```python
from build123d import *

# Parameters (mm, degrees)
SKETCH1_R           = 3.5
BOSS_EXTRUDE6_DEPTH = 5
CUT_EXTRUDE5_DEPTH  = 14.035691085
FILLET3_R           = 2
SKETCH3_R           = 3.5
BOSS_EXTRUDE9_DEPTH = 3


with BuildPart() as part:
    # Sketch1 → Boss-Extrude6 (new body)
    with BuildSketch(Plane.XY):
        with BuildLine():
            Line((1.138484568, -6.230529798), (82.159951164, -6.236480839))
            ThreePointArc((82.159951164, -6.236480839), (86.188937946, -4.567966564), (87.858044062, -0.539224931))
            Line((87.858044062, -0.539224931), (87.858163632, 1.088682041))
            ThreePointArc((87.858163632, 1.088682041), (86.189649357, 5.117668823), (82.160907724, 6.786774939))
            Line((82.160907724, 6.786774939), (8.344270935, 6.792196785))
            Line((8.344270935, 6.792196785), (-81.443742997, 6.79879173))
            ThreePointArc((-81.443742997, 6.79879173), (-85.472729779, 5.130277455), (-87.141835896, 1.101535822))
            Line((-87.141835896, 1.101535822), (-87.141955466, -0.52637115))
            ThreePointArc((-87.141955466, -0.52637115), (-85.473441191, -4.555357932), (-81.444699558, -6.224464049))
            Line((-81.444699558, -6.224464049), (1.138484568, -6.230529798))
        make_face()
        with Locations((82.160369659, 0)):
            Circle(SKETCH1_R, mode=Mode.SUBTRACT)
        with Locations((7.893112659, 0)):
            Circle(SKETCH1_R, mode=Mode.SUBTRACT)
    extrude(amount=BOSS_EXTRUDE6_DEPTH)

    # Sketch4 → Cut-Extrude5 (cut, through all)
    with BuildSketch(Plane(origin=(0.000498933, 6.792809636, 0), x_dir=(0.999999997, -7.345e-05, 0), z_dir=(7.345e-05, 0.999999997, 0))):
        Polygon((-97.188212117, 0), (-97.188212117, -3), (30.840558875, -3), (33.809433044, 0), align=None)
        Polygon((36.07564421, -2), (33.106770041, -5), (91.140577756, -5), (91.140577756, -2), align=None)
    extrude(amount=-CUT_EXTRUDE5_DEPTH, mode=Mode.SUBTRACT)

    # Fillet3
    fillet3_edges = [part.edges().sort_by_distance(p)[0] for p in [
        (33.809453605, 0.278698438, 0),
        (30.840579445, 0.278916502, 3),
        (33.106790605, 0.278750049, 5),
        (36.075664766, 0.278531984, 2),
    ]]
    fillet(fillet3_edges, radius=FILLET3_R)

    # Sketch3 → Boss-Extrude9 (add)
    with BuildSketch(Plane.XY.offset(5)):
        with Locations((-79.441895681, 0)):
            Circle(SKETCH3_R)
    extrude(amount=BOSS_EXTRUDE9_DEPTH)


solid = part.part
```
Check sheet for the modelled part. Datum: model origin and axes. Units: mm. A direction names the side the tool comes from. Round coordinates to 2 decimals unless told otherwise and drop trailing zeros. Write each loop counter-clockwise with the first axis right and the second up, starting at its lowest first coordinate (ties: lowest second). Pieces come first, ordered by that corner, then holes. Notation, with made-up numbers: M 13.5,-36 L 48.5,-36 A34 ccw 48.5,-4 Z; hole C 48.25,45 d1. An arc over 180 degrees is marked long. Write item = value, one per line. Start each with the question number.
1. Tool access check on faces 4 (the flat face through (-29, 0, 3)), 5 (the flat face through (-79, 0, 8)), 6 (the cylindrical face through (-76.21, -1.34, 6.48)). Record the directions out of +Z, -Z, +X, -X, +Y, -Y that give a thin tool (end or side, any length) a straight path to the whole face; none if there is none.
2. Section check A-A, the plane y = -2. State how many separate pieces and enclosed holes the cut face has, then the cut area to 3 significant figures.
3. Release check for a two-part mould opening along X. For faces 1 (the cylindrical face through (86.144, -4.612, 0.986)), 2 (the cylindrical face through (78.664, 0.154, 0.986)), 3 (the flat face through (63, 0, 2)) record: pulls with the +X half, pulls with the -X half, needs draft (parallel to the pull), parting line crosses it, or undercut.
4. Section check B-B, the plane x = 25.5. Record the cut outline in (y, z), then the cut area to 3 significant figures.
5. Scan lines: line 1 (Z direction, x = 26, y = 2); line 2 (Y direction, x = -36, z = 4); line 3 (X direction, y = -3, z = 1). Record each from-to range of solid material in increasing order. Write a range as [from, to].
6. Gauge pin test, flat ends, axial feed: pin 1 (4 mm diameter, centred on x = -50, y = 1.5, fed in from +Z); pin 2 (6.5 mm diameter, centred on x = -51.5, y = 3.5, fed in from -Z); pin 3 (2 mm diameter, centred on x = -21.5, z = 3.5, fed in from -Y); pin 4 (1 mm diameter, centred on x = 17, z = 1, fed in from -Y). Record the tip position at first contact, or that the pin passes through.
Results found:
q1.face_4 = -Z, -X, +Y, -Y
q1.face_5 = +Z, +X, -X, +Y, -Y
q1.face_6 = +Z
q2.separate_pieces = 3
q2.enclosed_holes = 0
q2.area = 350 mm^2
q3.face_1 = pulls with the +X half
q3.face_2 = undercut
q3.face_3 = needs draft
q4.outline = M -6.23,3 L 6.79,3 L 6.79,5 L -6.23,5 Z
q4.area = 26.0 mm^2
q5.line_1 = [3, 5]
q5.line_2 = [-6.23, 6.8]
q5.line_3 = [32.82, 80.36], [83.96, 87.3]
q6.pin_1 = 5
q6.pin_2 = 3
q6.pin_3 = -6.23
q6.pin_4 = through
